```python
from build123d import *

# Parameters (mm, degrees)
SKETCH_2_W          = 30
SKETCH_2_H          = 17
EXTRUDE_1_DEPTH     = 2
SKETCH_2_3_W        = 30
SKETCH_2_3_H        = 17
SKETCH_2_3_W_2      = 26
SKETCH_2_3_H_2      = 13
EXTRUDE_2_DEPTH     = 15
CUT_EXTRUDE_1_REACH = 29.185
SKETCH_3_W          = 23
SKETCH_3_H          = 12
CUT_EXTRUDE_2_REACH = 27.981
SKETCH_4_W          = 12
SKETCH_4_H          = 6
CHAMFER_2_SIZE      = 1
SKETCH_5_W          = 30
SKETCH_5_H          = 17
EXTRUDE_3_DEPTH     = 3
EXTRUDE_4_DEPTH     = 4
SKETCH_7_W          = 4
SKETCH_7_H          = 4
EXTRUDE_5_DEPTH     = 16
FILLET_1_R          = 2
CUT_EXTRUDE_3_DEPTH = 10


with BuildPart() as part:
    # 草图2 → 凸台-拉伸1 (new body)
    with BuildSketch(Plane(origin=(0, 0, 0), x_dir=(1, 0, 0), z_dir=(0, 1, 0))):
        Rectangle(SKETCH_2_W, SKETCH_2_H)
    extrude(amount=EXTRUDE_1_DEPTH)

    # 草图2<3> → 凸台-拉伸2 (add)
    with BuildSketch(Plane(origin=(0, 0, 0), x_dir=(1, 0, 0), z_dir=(0, 1, 0))):
        Rectangle(SKETCH_2_3_W, SKETCH_2_3_H)
        Rectangle(SKETCH_2_3_W_2, SKETCH_2_3_H_2, mode=Mode.SUBTRACT)
    extrude(amount=EXTRUDE_2_DEPTH)

    # 草图3 → 切除-拉伸1 (cut, up to next)
    with BuildSketch(Plane.XY.offset(8.5), mode=Mode.PRIVATE) as cut_extrude_1_sk1:
        with Locations((0, 9)):
            Rectangle(SKETCH_3_W, SKETCH_3_H)
    cut_extrude_1_tool1 = extrude(cut_extrude_1_sk1.sketch, amount=-CUT_EXTRUDE_1_REACH, mode=Mode.PRIVATE) & part.part
    add(cut_extrude_1_tool1.solids().sort_by_distance((0, 9, 8.5))[0], mode=Mode.SUBTRACT)

    # 草图4 → 切除-拉伸2 (cut, up to next)
    with BuildSketch(Plane.XY.offset(-6.5), mode=Mode.PRIVATE) as cut_extrude_2_sk1:
        with Locations((-7, 12)):
            Rectangle(SKETCH_4_W, SKETCH_4_H)
    cut_extrude_2_tool1 = extrude(cut_extrude_2_sk1.sketch, amount=-CUT_EXTRUDE_2_REACH, mode=Mode.PRIVATE) & part.part
    add(cut_extrude_2_tool1.solids().sort_by_distance((-7, 12, -6.5))[0], mode=Mode.SUBTRACT)

    # 倒角2
    chamfer_2_edges = [part.edges().sort_by_distance(p)[0] for p in [
        (13, 15, 0),
        (6, 15, -6.5),
        (-13, 15, -1),
        (-12.25, 15, 6.5),
        (12.25, 15, 6.5),
    ]]
    chamfer(chamfer_2_edges, length=CHAMFER_2_SIZE)

    # 草图5 → 凸台-拉伸3 (add)
    with BuildSketch(Plane.XZ):
        Rectangle(SKETCH_5_W, SKETCH_5_H)
    extrude(amount=EXTRUDE_3_DEPTH)

    # 草图6 → 凸台-拉伸4 (add)
    with BuildSketch(Plane.XZ.offset(3)):
        Polygon((-12.5, -3.5), (-10.5, -3.5), (-10.5, -8.5), (-14.5, -8.5), (-14.5, -3.5), align=None)
    extrude_4 = extrude(amount=EXTRUDE_4_DEPTH)

    # 草图7 → 凸台-拉伸5 (add)
    with BuildSketch(Plane(origin=(0, 0, -8.5), x_dir=(-1, 0, 0), z_dir=(0, 0, -1))):
        with Locations((12.5, -9)):
            Rectangle(SKETCH_7_W, SKETCH_7_H)
    extrude_5 = extrude(amount=-EXTRUDE_5_DEPTH)

    # 镜向1: 凸台-拉伸4, 凸台-拉伸5 across plane
    add(extrude_4.mirror(Plane(origin=(0, 0, 0), x_dir=(0, 0, 1), z_dir=(1, 0, 0))))
    add(extrude_5.mirror(Plane(origin=(0, 0, 0), x_dir=(0, 0, 1), z_dir=(1, 0, 0))))

    # 圆角1
    fillet_1_edges = [part.edges().sort_by_distance(p)[0] for p in [
        (-12.5, -7, -3.5),
        (12.5, -7, -3.5),
    ]]
    fillet(fillet_1_edges, radius=FILLET_1_R)

    # 草图8 → 切除-拉伸3 (cut)
    with BuildSketch(Plane(origin=(0, 15, 0), x_dir=(1, 0, 0), z_dir=(0, 1, 0))):
        Polygon((13, 6.5), (13, 9.517493256), (-13, 9.517493256), (-13, 5.799908087), (12.835608811, 5.799908087), align=None)
    extrude(amount=-CUT_EXTRUDE_3_DEPTH, mode=Mode.SUBTRACT)


solid = part.part
```
CAD build for the part. Positions are in the model's coordinates, mm. A direction names the side the tool comes from. Round coordinates to 2 decimals unless told otherwise and drop trailing zeros. Order: outer loops, then holes, each group sorted by start corner. A loop starts at its lowest first (then second) coordinate and runs counter-clockwise, first axis right, second up. Notation, with made-up numbers: (36.25, 32.5) - (67.25, 32.5) arc R8 cw to (67.25, 37.5) - close; hole circle Ø11 at (49.5, 60.25). An arc over 180 degrees is marked (long way). Use CSV: the item, a comma, the result in double quotes. Start each with the question number.
1) Saw through at C-C (x = -12). List the corners of the cut face in (y, z), and give its area (3 significant figures).
2) Saw through at B-B (z = -0.25). List the corners of the cut face in (x, y), and give its area (3 significant figures).
3) Saw through at A-A (y = 12). List the corners of the cut face in (x, z).
4) Pin check, flat tips, straight feed: pin 1 Ø1.2 at (x, z) = (-12.5, 2) entering from +Y; pin 2 Ø2.5 at (y, z) = (-9, -0.5) entering from +X; pin 3 Ø5 at (x, z) = (1.5, -4) entering from -Y; pin 4 Ø2 at (x, y) = (-0.5, -5) entering from -Z. Stop position of each tip, or through.
5) Saw through at D-D (y = -8). List the corners of the cut face in (x, z), and give its area (3 significant figures).
6) Wall check: L1, parallel to X at y = 13.5, z = -1.5; L2, parallel to X at y = -8.25, z = 1.25; L3, parallel to Z at x = -4, y = 2.25. Give the ranges that are in metal, low to high. Write a range as [from, to].
7) Two-plate mould, pull along X, no slides. Class faces 1 (the flat face through (0, 3, -6.5)), 2 (the flat face through (0, 2, 8.5)), 3 (the flat face through (14.5, -8, -2)): pulls with the +X half, pulls with the -X half, needs draft (parallel to the pull), parting line crosses it, or undercut.
8) Tool access for faces 4 (the flat face through (-10.5, -8, -2)), 5 (the flat face through (-2.9, 2.6, 6.5)), 6 (the flat face through (0, -3, 0)), 7 (the flat face through (-13.5, 14.5, -0.4)), 8 (the flat face through (12, -9, 7.5)): list every direction of +Z, -Z, +X, -X, +Y, -Y with a clear straight run to the whole face (end or side of a thin tool).
Values follow:
1,outline,"(-11, -8.5) - (5, -8.5) - (5, -6.5) - (2, -6.5) - (2, 6.5) - (14, 6.5) - (15, 7.5) - (15, 8.5) - (-3, 8.5) - (-3, -3.5) - (-5, -3.5) arc R2 cw to (-7, -1.5) - (-7, 7.5) - (-11, 7.5) - close"
1,area,"201 mm2"
2,outline,"(-15, -3) - (15, -3) - (15, 15) - (14, 15) - (13, 14) - (13, 2) - (-13, 2) - (-13, 14) - (-14, 15) - (-15, 15) - close; (-14.5, -11) - (-10.5, -11) - (-10.5, -7) - (-14.5, -7) - close; (10.5, -11) - (14.5, -11) - (14.5, -7) - (10.5, -7) - close"
2,area,"233 mm2"
3,outline,"(-15, -8.5) - (-13, -8.5) - (-13, 6.5) - (-11.5, 6.5) - (-11.5, 8.5) - (-15, 8.5) - close; (11.5, 6.5) - (13, 6.5) - (13, -8.5) - (15, -8.5) - (15, 8.5) - (11.5, 8.5) - close"
4,pin 1,"stops at y = 14.1"
4,pin 2,"stops at x = 14.5"
4,pin 3,"stops at y = -3"
4,pin 4,"passes through"
5,outline,"(-14.5, -8.5) - (-10.5, -8.5) - (-10.5, 7.5) - (-14.5, 7.5) - close; (10.5, -8.5) - (14.5, -8.5) - (14.5, 7.5) - (10.5, 7.5) - close"
5,area,"128 mm2"
6,L1,"x = [-15, -13], [13, 15]"
6,L2,"x = [-14.5, -10.5], [10.5, 14.5]"
6,L3,"z = [-8.5, -6.5], [6.5, 8.5]"
7,face 1,"undercut"
7,face 2,"needs draft"
7,face 3,"pulls with the +X half"
8,face 4,"+Z, -Z, -Y"
8,face 5,"+Y"
8,face 6,"+Z"
8,face 7,"-Z, +Y"
8,face 8,"+Z, +X, -X, -Y"
